Here's how the part is built. I have some questions about the finished solid (model axes, mm). Coordinates: 2 decimals unless noted, no trailing zeros. Write each loop counter-clockwise with the first axis right and the second up, starting at its lowest first coordinate (ties: lowest second). Pieces come first, ordered by that corner, then holes.
Item 1: If we section it at C-C (x = -18): Please give me the cut outline in (y, z), then the cut area to 3 significant figures.
Item 2: If we section it at B-B (y = -42): Please give me the cut outline in (x, z), then the cut area to 3 significant figures.
Item 3: If I drill on line 1 (Y direction, x = -21.92, z = 0.9); line 2 (Y direction, x = -18, z = 0.55), over which ranges is the centre line in solid material (lowest first)?
Item 4: If we section it at D-D (z = 1.3): Count the separate pieces of the cut face and the enclosed holes in it, then the cut area to 3 significant figures.
Item 5: If we section it at A-A (x = 0): Please give me the cut outline in (y, z), then the cut area to 3 significant figures.
from build123d import *

# Parameters (mm, degrees)
F0_R     = 1.2
F0_R_2   = 2.5
F0_R_3   = 1.5
F1_DEPTH = 2
F2_R     = 10
F3_R     = 8


with BuildPart() as f1:
    # F0 (on Top) → F1 (new body)
    with BuildSketch(Plane.XY):
        with BuildLine():
            ThreePointArc((-5.2915026221, 6), (0, 8), (5.2915026221, 6))
            Line((5.2915026221, 6), (16.9705627485, 6))
            ThreePointArc((16.9705627485, 6), (0, 18), (-16.9705627485, 6))
            Line((-16.9705627485, 6), (-5.2915026221, 6))
        make_face()
        with BuildLine():
            ThreePointArc((5.2915026221, 6), (7.2915026221, 3.2915026221), (8, 0))
            ThreePointArc((8, 0), (-3.2915026221, -7.2915026221), (-5.2915026221, 6))
            Line((-5.2915026221, 6), (-16.9705627485, 6))
            ThreePointArc((-16.9705627485, 6), (-3.0438356171, -17.7407740738), (18, 0))
            ThreePointArc((18, 0), (17.7407740738, 3.0438356171), (16.9705627485, 6))
            Line((16.9705627485, 6), (5.2915026221, 6))
        make_face()
        with Locations((-13.55, 0)):
            Circle(F0_R, mode=Mode.SUBTRACT)
        with Locations((13.55, 0)):
            Circle(F0_R, mode=Mode.SUBTRACT)
        with BuildLine():
            Line((25.5, 6), (16.9705627485, 6))
            ThreePointArc((16.9705627485, 6), (17.7407740738, 3.0438356171), (18, 0))
            ThreePointArc((18, 0), (-3.0438356171, -17.7407740738), (-16.9705627485, 6))
            Line((-16.9705627485, 6), (-25.5, 6))
            Line((-25.5, 6), (-25.5, -52))
            Line((-25.5, -52), (25.5, -52))
            Line((25.5, -52), (25.5, 6))
        make_face()
        with Locations((-18, -42)):
            Circle(F0_R_2, mode=Mode.SUBTRACT)
        with Locations((18, -42)):
            Circle(F0_R_2, mode=Mode.SUBTRACT)
        with Locations((-21.92, 0)):
            Circle(F0_R_3, mode=Mode.SUBTRACT)
        with Locations((21.92, 0)):
            Circle(F0_R_3, mode=Mode.SUBTRACT)
    extrude(amount=F1_DEPTH)

    # F2
    f2_edges = [f1.edges().sort_by_distance(p)[0] for p in [
        (-16.970563, 6, 1),
        (16.970563, 6, 1),
    ]]
    fillet(f2_edges, radius=F2_R)

    # F3
    f3_edges = [f1.edges().sort_by_distance(p)[0] for p in [
        (25.5, 6, 1),
        (-25.5, 6, 1),
    ]]
    fillet(f3_edges, radius=F3_R)


solid = f1.part
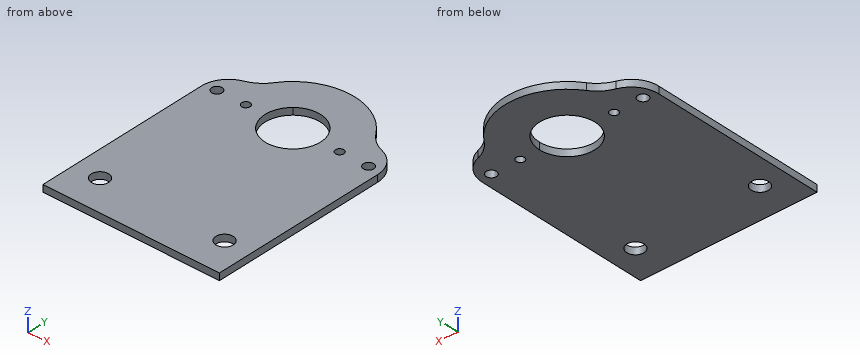
Answer list:
1. outline: (-52, 0) - (-44.5, 0) - (-44.5, 2) - (-52, 2) - close; (-39.5, 0) - (7.33, 0) - (7.33, 2) - (-39.5, 2) - close
1. area: 109 mm2
2. outline: (-25.5, 0) - (-20.5, 0) - (-20.5, 2) - (-25.5, 2) - close; (-15.5, 0) - (15.5, 0) - (15.5, 2) - (-15.5, 2) - close; (20.5, 0) - (25.5, 0) - (25.5, 2) - (20.5, 2) - close
2. area: 82.0 mm2
3. line 1: y = -52 to -1.5, 1.5 to 5.52
3. line 2: y = -52 to -44.5, -39.5 to 7.33
4. separate pieces: 1
4. enclosed holes: 7
4. area: 2,980 mm2
5. outline: (-52, 0) - (-8, 0) - (-8, 2) - (-52, 2) - close; (8, 0) - (18, 0) - (18, 2) - (8, 2) - close
5. area: 108 mm2
